Geometry check sheet. Reference: drawing and pictorial views, mm from the part's lowest x, y, z. A direction names the side the tool comes from. Give positions to 0.01 mm unless a question says otherwise; leave off trailing zeros. Order: outer loops, then holes, each group sorted by start corner. A loop starts at its lowest first (then second) coordinate and runs counter-clockwise, first axis right, second up. Notation, with made-up numbers: (-23.75, 36.25) -> (33.25, 36.25) arc R21 cw to (33.25, 46.25) -> close; hole circle Ø4 at (-35.5, -36). An arc over 180 degrees is marked (long way). Write each question's results on one line, items separated by ' | '.
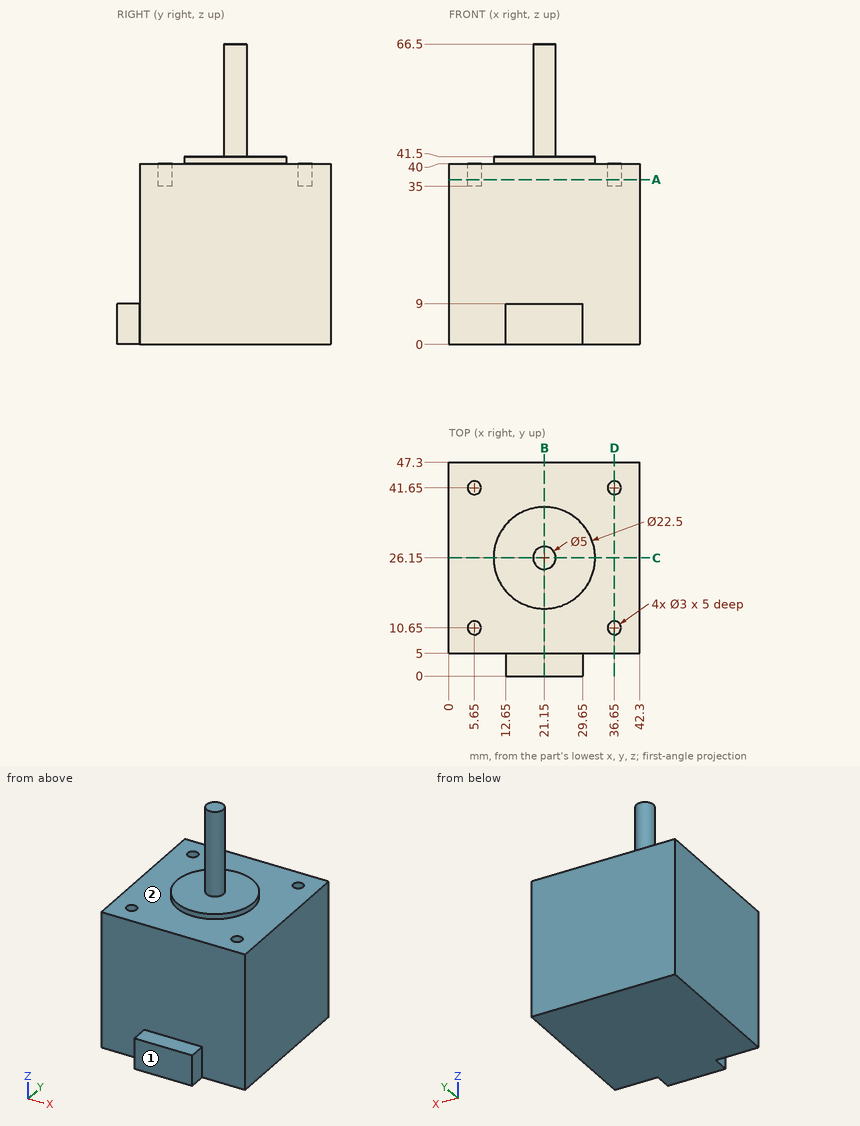
1. Section check B-B on x = 21.15. Record the cut outline in (y, z), then the cut area to 3 significant figures.
Verdict:
outline: (0, 0) -> (47.3, 0) -> (47.3, 40) -> (37.4, 40) -> (37.4, 41.5) -> (28.65, 41.5) -> (28.65, 66.5) -> (23.65, 66.5) -> (23.65, 41.5) -> (14.9, 41.5) -> (14.9, 40) -> (5, 40) -> (5, 9) -> (0, 9) -> close | area: 1,900 mm^2
2. Material ranges on probe 1 along Y at (x, z) = (5.65, 38.2); probe 2 along X at (y, z) = (10, 36); probe 3 along Y at (x, z) = (5, 37), recorded low to high. Write a range as from..to.
Verdict:
probe 1: y = 5..9.15, 12.15..40.15, 43.15..47.3 | probe 2: x = 0..4.3, 7..35.3, 38..42.3 | probe 3: y = 5..9.3, 12..40.3, 43..47.3
3. Gauge pin test, flat ends, axial feed: pin 1 Ø3 at (x, y) = (9, 31) entering from -Z; pin 2 Ø5.5 at (x, y) = (17.5, 1.5) entering from +Z; pin 3 Ø2.5 at (y, z) = (3.5, 5.5) entering from +X; pin 4 Ø3.5 at (x, y) = (36.5, 41) entering from +Z. Record the tip position at first contact, or that the pin passes through.
Verdict:
pin 1: stops at z = 0 | pin 2: stops at z = 9 | pin 3: stops at x = 29.65 | pin 4: stops at z = 40
4. Access from +Z, -Z, +X, -X, +Y, -Y to the whole of each face (thin tool, end or side, straight path). Record for the marked faces 1 and 2.
Verdict:
face 1: +Z, -Z, +X, -X, -Y | face 2: +Z
5. Section check D-D on x = 36.65. Record the cut outline in (y, z).
Verdict:
outline: (5, 0) -> (47.3, 0) -> (47.3, 40) -> (43.15, 40) -> (43.15, 35) -> (40.15, 35) -> (40.15, 40) -> (12.15, 40) -> (12.15, 35) -> (9.15, 35) -> (9.15, 40) -> (5, 40) -> close
6. Section check C-C on y = 26.15. Record the cut outline in (x, z), then the cut area to 3 significant figures.
Verdict:
outline: (0, 0) -> (42.3, 0) -> (42.3, 40) -> (32.4, 40) -> (32.4, 41.5) -> (23.65, 41.5) -> (23.65, 66.5) -> (18.65, 66.5) -> (18.65, 41.5) -> (9.9, 41.5) -> (9.9, 40) -> (0, 40) -> close | area: 1,850 mm^2
7. Section check A-A on z = 36.5. Record the cut outline in (x, y).
Verdict:
outline: (0, 5) -> (42.3, 5) -> (42.3, 47.3) -> (0, 47.3) -> close; hole circle Ø3 at (5.65, 10.65); hole circle Ø3 at (5.65, 41.65); hole circle Ø3 at (36.65, 10.65); hole circle Ø3 at (36.65, 41.65)
